from build123d import *

# Parameters (mm, degrees)
F1_DEPTH = 508
F2_W     = 80.340108
F2_H     = 50.8
F2_W_2   = 82.870346
F3_DEPTH = 19.05


with BuildPart() as f1:
    # F0 (on Front) → F1 (new body)
    with BuildSketch(Plane.XZ):
        with BuildLine():
            Line((3.550242, 42.501207), (-21.849758, 42.501207))
            ThreePointArc((-21.849758, 42.501207), (-32.272509, 23.451207), (-21.849758, 4.401207))
            Line((-21.849758, 4.401207), (3.550242, 4.401207))
            ThreePointArc((3.550242, 4.401207), (13.712078, 23.451207), (3.550242, 42.501207))
        make_face()
    extrude(amount=F1_DEPTH)

    # F2 (on face) → F3 (cut)
    with BuildSketch(Plane.XY.offset(42.501207)):
        with Locations((-9.149758, -406.4)):
            Rectangle(F2_W, F2_H)
        with Locations((-9.149758, -101.6)):
            Rectangle(F2_W_2, F2_H)
    extrude(amount=-F3_DEPTH, mode=Mode.SUBTRACT)


solid = f1.part
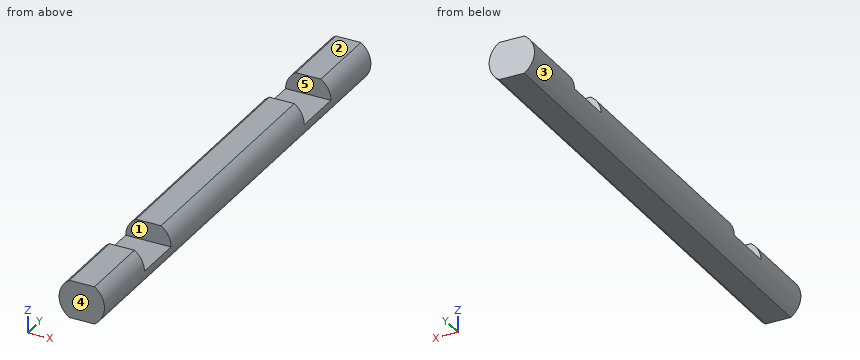
Could you check a few things on this model? Use its own coordinates, in mm. Face numbers are marked on the shaded views. A direction names the side the tool comes from. Give positions to 0.01 mm unless a question says otherwise; leave off trailing zeros. Order: outer loops, then holes, each group sorted by start corner. A loop starts at its lowest first (then second) coordinate and runs counter-clockwise, first axis right, second up. Notation, with made-up numbers: (-13.5, 29.25) - (14.5, 29.25) arc R25 ccw to (14.5, 48.25) - close; hole circle Ø4 at (-30, 70.25). An arc over 180 degrees is marked (long way). One line per question, with ' | ' between items. Start each with the question number.
Item 1: I want a section at A-A on x = -3.5. Write out the boundary of the cut face in (y, z), then the cut area to 3 significant figures.
Item 2: I want a section at C-C on y = -103.5. Write out the boundary of the cut face in (x, z).
Item 3: Thinking about a two-plate mould opening in Y: for the marked faces 3, 4 and 5, which applies, pulls with the +Y half, pulls with the -Y half, needs draft (parallel to the pull), parting line crosses it, or undercut?
Item 4: I'm going to push flat-ended pins straight in: pin 1 Ø4 at (x, y) = (8.5, -258) entering from -Z; pin 2 Ø23 at (x, y) = (-5, -101.5) entering from +Z; pin 3 Ø2 at (y, z) = (-249, 29.5) entering from -X. Where does each tip first touch, or does it pass through?
Item 5: I need wall thicknesses on probe 1 along Y at (x, z) = (-0.5, 30.5); probe 2 along Z at (x, y) = (-12, -424.5); probe 3 along X at (y, z) = (-324.5, 21.5). Which ranges of each line are inside material? Lowest first, please. Write a range as [from, to].
Item 6: I want a section at D-D on y = -199.5. Write out the boundary of the cut face in (x, z).
Item 7: For the marked faces 1 and 2, which set-ups out of +Z, -Z, +X, -X, +Y, -Y let a thin tool reach every point of the face, with its end or its side?
Item 8: I want a section at B-B on z = 34. Write out the boundary of the cut face in (x, y), then the cut area to 3 significant figures.
Verdict:
1) outline: (-508, 4.4) - (0, 4.4) - (0, 42.5) - (-76.2, 42.5) - (-76.2, 23.45) - (-127, 23.45) - (-127, 42.5) - (-381, 42.5) - (-381, 23.45) - (-431.8, 23.45) - (-431.8, 42.5) - (-508, 42.5) - close | area: 17,400 mm^2
2) outline: (-32.27, 23.45) arc R22.62 ccw to (-21.85, 4.4) - (3.55, 4.4) arc R22.94 ccw to (13.71, 23.45) - close
3) face 3: needs draft | face 4: pulls with the -Y half | face 5: undercut
4) pin 1: z = 6.75 | pin 2: z = 23.45 | pin 3: x = -31.7
5) probe 1: [-508, -431.8], [-381, -127], [-76.2, 0] | probe 2: [4.4, 23.45] | probe 3: [-32.19, 13.63]
6) outline: (-21.85, 4.4) - (3.55, 4.4) arc R22.94 ccw to (3.55, 42.5) - (-21.85, 42.5) arc R22.62 ccw to start
7) face 1: +Z, +X, -X | face 2: +Z, +X, -X, +Y, -Y
8) outline: (-29.66, -508) - (11.14, -508) - (11.14, -431.8) - (-29.66, -431.8) - close; (-29.66, -381) - (11.14, -381) - (11.14, -127) - (-29.66, -127) - close; (-29.66, -76.2) - (11.14, -76.2) - (11.14, 0) - (-29.66, 0) - close | area: 16,600 mm^2
